Model file for the job. Use its own axes, mm. Face numbers are marked on the shaded views. A direction names the side the tool comes from. Give positions to 0.01 mm unless a question says otherwise; leave off trailing zeros. Write each loop counter-clockwise with the first axis right and the second up, starting at its lowest first coordinate (ties: lowest second). Pieces come first, ordered by that corner, then holes.
```python
from build123d import *

# Parameters (mm, degrees)
F0_R     = 4
F1_DEPTH = 50
F3_DEPTH = 5
F4_R     = 1.5
F5_DEPTH = 5


with BuildPart() as f1:
    # F0 (on Top) → F1 (new body)
    with BuildSketch(Plane.XY):
        Circle(F0_R)
    extrude(amount=F1_DEPTH)

    # F2 (on face) → F3 (join)
    with BuildSketch(Plane.XY.offset(50)):
        Polygon((6.928004, -0.052545), (3.509508, 5.973555), (-3.418496, 6.0261), (-6.928004, 0.052545), (-3.509508, -5.973555), (3.418496, -6.0261), align=None)
    extrude(amount=F3_DEPTH)

    # F4 (on face) → F5 (join)
    with BuildSketch(Plane.XY.offset(55)):
        Circle(F4_R)
    extrude(amount=F5_DEPTH)

    # F6 (on Front) → F7 (revolve)
    with BuildSketch(Plane.XZ):
        with BuildLine():
            Line((-15, 65), (-15, 62))
            ThreePointArc((-15, 62), (-8.276473, 56.83613), (0, 55))
            Line((0, 55), (0, 65))
            Line((0, 65), (-15, 65))
        make_face()
    revolve(axis=Axis((0, 0, 60), (0, 0, -1)))


solid = f1.part
```
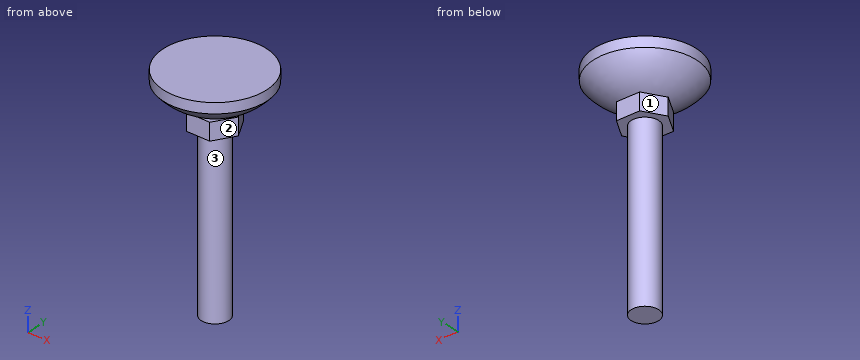
1. Pin check, flat tips, straight feed: P1, Ø2, axis at y = 2, z = 27.5, coming from the +X side; P2, Ø10, axis at x = -11, z = 54.5, coming from the +Y side; P3, Ø12, axis at x = -11, z = 54, coming from the +Y side. Stop position of each tip, or through.
Calculated:
P1: stops at x = 3.87
P2: stops at y = 7.94
P3: stops at y = 9.1
2. Which spindle directions (+Z, -Z, +X, -X, +Y, -Y) get a long thin tool onto all of the face, cutting with end or side? Do the marked faces 1, 2 and 3. Say none if no direction does.
Calculated:
face 1: -Z, -X, +Y
face 2: -Z, +X, -Y
face 3: -Z
3. Slice it at A-A, the plane z = 53.5. Write the cut outline in (x, y).
Calculated:
outline: (-6.93, 0.05) - (-3.51, -5.97) - (3.42, -6.03) - (6.93, -0.05) - (3.51, 5.97) - (-3.42, 6.03) - close
4. Probe probe 1 along Z at (x, y) = (2, 3); probe 2 along Z at (x, y) = (7, -9.5); probe 3 along Z at (x, y) = (10, 3). List the from-to ranges inside material, lowest first.
Calculated:
probe 1: z = 0 to 55, 55.33 to 65
probe 2: z = 58.96 to 65
probe 3: z = 58.02 to 65
5. Slice it at B-B, the plane z = 7.5. Write the cut outline in (x, y).
Calculated:
outline: circle Ø8 at (0, 0)
